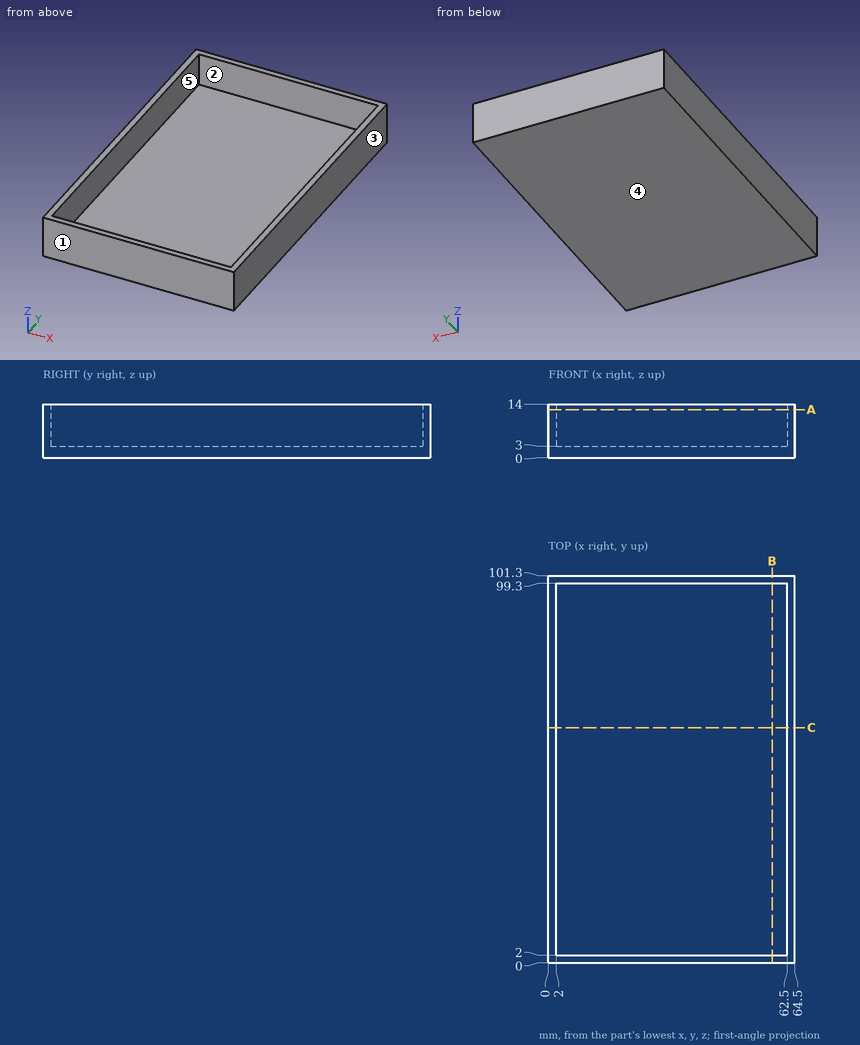
Geometry: see drawing. Coordinates: mm, zero at the bounding-box minimum. A direction names the side the tool comes from. Coordinates: 2 decimals unless noted, no trailing zeros. Loops run counter-clockwise (first coordinate to the right, second up) from the corner with the lowest first, then second, coordinate; pieces in that order, holes last. Notation, with made-up numbers: (50.25, 68.5) - (96.25, 68.5) arc R21 cw to (96.25, 90.5) - close; hole circle Ø2 at (38.25, 31.25). An arc over 180 degrees is marked (long way). Answer in a Markdown table with one row per item.
(1) Cut plane A-A on z = 12.5. Output: boundary loops of the cut face in (x, y), plus the area to 3 significant figures.
Model answer:
| item | result |
|---|---|
| outline | (0, 0) - (64.5, 0) - (64.5, 101.3) - (0, 101.3) - close; hole (2, 2) - (62.5, 2) - (62.5, 99.3) - (2, 99.3) - close |
| area | 647 mm² |
(2) Cut plane B-B on x = 58.5. Output: boundary loops of the cut face in (y, z).
Model answer:
| item | result |
|---|---|
| outline | (0, 0) - (101.3, 0) - (101.3, 14) - (99.3, 14) - (99.3, 3) - (2, 3) - (2, 14) - (0, 14) - close |
(3) Mould query, pull axis X, two halves, no side actions, for the marked faces 1, 2 and 3. Classes: pulls with the +X half, pulls with the -X half, needs draft (parallel to the pull), parting line crosses it, or undercut.
Model answer:
| item | result |
|---|---|
| face 1 | needs draft |
| face 2 | undercut |
| face 3 | pulls with the +X half |
(4) Set-up query: the marked faces 4 and 5. Return all of +Z, -Z, +X, -X, +Y, -Y with unobstructed straight access to the full face (end or side cutting, diameter ignored); none if empty.
Model answer:
| item | result |
|---|---|
| face 4 | -Z, +X, -X, +Y, -Y |
| face 5 | +Z |
(5) Cut plane C-C on y = 61.5. Output: boundary loops of the cut face in (x, z), plus the area to 4 significant figures.
Model answer:
| item | result |
|---|---|
| outline | (0, 0) - (64.5, 0) - (64.5, 14) - (62.5, 14) - (62.5, 3) - (2, 3) - (2, 14) - (0, 14) - close |
| area | 237.5 mm² |
(6) Material intervals for L1, parallel to X at y = 67, z = 4.5; L2, parallel to Y at x = 15.5, z = 12; L3, parallel to Z at x = 60.5, y = 19, sorted ascending. Write a range as from..to.
Model answer:
| item | result |
|---|---|
| L1 | x = 0..2, 62.5..64.5 |
| L2 | y = 0..2, 99.3..101.3 |
| L3 | z = 0..3 |
(7) Pin query (flat end, axial travel): P1, Ø12, axis at x = 55, y = 30.5, coming from the +Z side. Return the tip coordinate at first contact, or that it passes through.
Model answer:
| item | result |
|---|---|
| P1 | stops at z = 3 |
